```python
from build123d import *

# Parameters (mm, degrees)
EXTRUDE_1_DEPTH     = 20
CUT_EXTRUDE_1_DEPTH = 149.381528207
CUT_EXTRUDE_2_DEPTH = 154.011402085


with BuildPart() as part:
    # Эскиз1 → Бобышка-Вытянуть1 (new body)
    with BuildSketch(Plane.XY):
        Polygon((0, 0), (0, -8), (100, -8), (121.213203436, 13.213203436), (121.213203436, 83.213203436), (113.213203436, 83.213203436), (113.213203436, 16.526911935), (96.686291501, 0), align=None)
    extrude(amount=EXTRUDE_1_DEPTH)

    # Эскиз2 → Вырез-Вытянуть1 (cut, through all)
    with BuildSketch(Plane.ZY):
        Polygon((0, -3), (2.886751346, -3), (0, -8), align=None)
        Polygon((20, -8), (20, -3), (17.113248654, -3), align=None)
    extrude(amount=-CUT_EXTRUDE_1_DEPTH, mode=Mode.SUBTRACT)

    # Эскиз3 → Вырез-Вытянуть2 (cut, through all)
    with BuildSketch(Plane(origin=(0, 83.213203436, 0), x_dir=(1, 0, 0), z_dir=(0, 1, 0))):
        Polygon((116.213203436, -20), (116.213203436, -17.113248654), (121.213203436, -20), align=None)
        Polygon((121.213203436, 0), (116.213203436, 0), (116.213203436, -2.886751346), align=None)
    extrude(amount=-CUT_EXTRUDE_2_DEPTH, mode=Mode.SUBTRACT)


solid = part.part
```
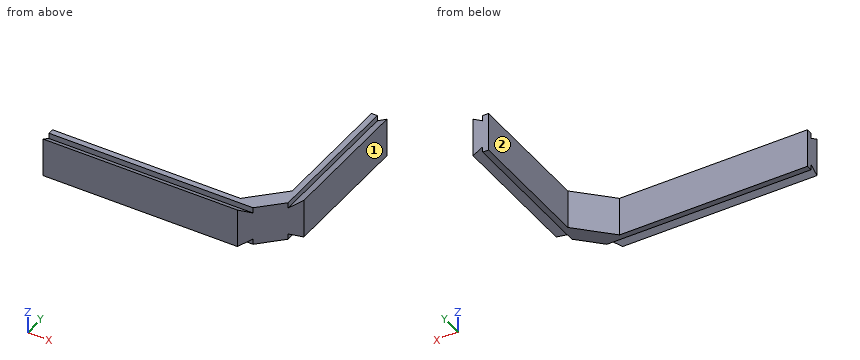
Read the model definition and answer for the solid it produces. Units are mm, in the model's axes. Face numbers are marked on the shaded views. A direction names the side the tool comes from. Coordinates: 2 decimals unless noted, no trailing zeros. Loops run counter-clockwise (first coordinate to the right, second up) from the corner with the lowest first, then second, coordinate; pieces in that order, holes last. Notation, with made-up numbers: (65, -37) - (115, -37) arc R33 ccw to (115, -8) - close; hole circle Ø5 at (-13.5, 19.25). An arc over 180 degrees is marked (long way). Answer in a Markdown table with one row per item.
1. Straight lines are drawn through the part: line 1 (Y direction, x = 85, z = 4.5); line 2 (X direction, y = 14.5, z = 2.5); line 3 (Y direction, x = 37, z = 18.5). For each, find the intervals that lie inside material, in ascending order.
Conclusion:
| item | result |
|---|---|
| line 1 | y = -8 to 0 |
| line 2 | x = 111.19 to 116.21, 116.88 to 121.21 |
| line 3 | y = -8 to -5.4, -3 to 0 |
2. Find section B-B, the plane z = 15.5. Write down the section's boundary in (x, y).
Conclusion:
| item | result |
|---|---|
| outline | (0, -8) - (100, -8) - (121.21, 13.21) - (121.21, 83.21) - (113.21, 83.21) - (113.21, 16.53) - (96.69, 0) - (0, 0) - close |
3. Given pin 1 (10 mm diameter, centred on y = 45.5, z = 8, fed in from -X); pin 2 (12 mm diameter, centred on y = 8.5, z = 15, fed in from -X), each flat-ended and moving along its own axis, determine where each tip first touches the part or whether it passes through.
Conclusion:
| item | result |
|---|---|
| pin 1 | stops at x = 113.21 |
| pin 2 | stops at x = 99.19 |
4. Which of the six approach directions +Z, -Z, +X, -X, +Y, -Y give full straight-line access (tool end or side, diameter ignored) to the marked faces 1 and 2?
Conclusion:
| item | result |
|---|---|
| face 1 | +Z, -Z, +X, +Y, -Y |
| face 2 | +Z, -Z, -X, +Y |
5. Find section D-D, the plane x = 107. Write down the section's boundary in (y, z), then the cut area to 3 significant figures.
Conclusion:
| item | result |
|---|---|
| outline | (-1, 0) - (10.31, 0) - (10.31, 20) - (-1, 20) - close |
| area | 226 mm² |
6. Find section C-C, the plane z = 1.5. Write down the section's boundary in (x, y), then the cut area to 3 significant figures.
Conclusion:
| item | result |
|---|---|
| outline | (0, -8) - (100, -8) - (102.6, -5.4) - (0, -5.4) - close; (0, -3) - (105, -3) - (116.21, 8.21) - (116.21, 83.21) - (113.21, 83.21) - (113.21, 16.53) - (96.69, 0) - (0, 0) - close; (118.62, 10.62) - (121.21, 13.21) - (121.21, 83.21) - (118.62, 83.21) - close |
| area | 1,120 mm² |
7. Find section A-A, the plane y = 51. Write down the section's boundary in (x, z).
Conclusion:
| item | result |
|---|---|
| outline | (113.21, 0) - (116.21, 0) - (116.21, 2.89) - (121.21, 0) - (121.21, 20) - (116.21, 17.11) - (116.21, 20) - (113.21, 20) - close |
